```python
from build123d import *

# Parameters (mm, degrees)
SKETCH1_R                       = 12.7
BOSS_EXTRUDE1_DEPTH             = 25.4
CUT_EXTRUDE1_DEPTH              = 333.148099498
CUT_EXTRUDE1_DEPTH_BACK         = 333.148099498
SKETCH2_W                       = 25.4
SKETCH2_H                       = 50.8
BOSS_EXTRUDE2_REACH             = 334.148
SKETCH1_2_R                     = 12.7
BOSS_EXTRUDE2_DIRECTION_2_REACH = 334.148


with BuildPart() as part:
    # Sketch1 → Boss-Extrude1 (new, symmetric)
    with BuildSketch(Plane.XY):
        with BuildLine():
            Line((-25.4, 0), (-25.4, 304.8))
            ThreePointArc((-25.4, 304.8), (0, 330.2), (25.4, 304.8))
            Line((25.4, 304.8), (25.4, 0))
            ThreePointArc((25.4, 0), (0, -25.4), (-25.4, 0))
        make_face()
        Circle(SKETCH1_R, mode=Mode.SUBTRACT)
        with Locations((0, 304.8)):
            Circle(SKETCH1_R, mode=Mode.SUBTRACT)
    extrude(amount=BOSS_EXTRUDE1_DEPTH, both=True)

    # Sketch2 → Cut-Extrude1 (cut, two sides: drawn at the far end of the back side and taken through both)
    with BuildSketch(Plane(origin=(0, 0, 0), x_dir=(0, 0, -1), z_dir=(1, 0, 0)).offset(-CUT_EXTRUDE1_DEPTH_BACK)):
        with Locations((0, 304.8)):
            Rectangle(SKETCH2_W, SKETCH2_H)
        Rectangle(SKETCH2_W, SKETCH2_H)
    extrude(amount=CUT_EXTRUDE1_DEPTH + CUT_EXTRUDE1_DEPTH_BACK, mode=Mode.SUBTRACT)

    # Boss-Extrude2: up to this face of the body (flat: up to its plane)
    boss_extrude2_end = Plane(part.part.faces().sort_by_distance((0, 152.4, -25.4))[0])
    # Sketch1<2> → Boss-Extrude2 (add, up to the picked face)
    with BuildSketch(Plane.XY, mode=Mode.PRIVATE) as boss_extrude2_sk1:
        Circle(SKETCH1_2_R)
    boss_extrude2_tool1 = split(extrude(boss_extrude2_sk1.sketch, amount=-BOSS_EXTRUDE2_REACH, mode=Mode.PRIVATE), bisect_by=boss_extrude2_end, keep=Keep.BOTH, mode=Mode.PRIVATE)
    # Sketch1<2> → Boss-Extrude2 (add, up to the picked face)
    with BuildSketch(Plane.XY, mode=Mode.PRIVATE) as boss_extrude2_sk2:
        with Locations((0, 304.8)):
            Circle(SKETCH1_2_R)
    boss_extrude2_tool2 = split(extrude(boss_extrude2_sk2.sketch, amount=-BOSS_EXTRUDE2_REACH, mode=Mode.PRIVATE), bisect_by=boss_extrude2_end, keep=Keep.BOTH, mode=Mode.PRIVATE)
    add(boss_extrude2_tool1.solids().sort_by(Axis((0, 0, 0), (0, 0, -1)))[0])
    add(boss_extrude2_tool2.solids().sort_by(Axis((0, 304.8, 0), (0, 0, -1)))[0])

    # Boss-Extrude2 direction 2: up to this face of the body (flat: up to its plane)
    boss_extrude2_direction_2_end = Plane(part.part.faces().sort_by_distance((0, 152.4, 25.4))[0])
    # Sketch1<2> → Boss-Extrude2 direction 2 (add, up to the picked face)
    with BuildSketch(Plane.XY, mode=Mode.PRIVATE) as boss_extrude2_direction_2_sk1:
        Circle(SKETCH1_2_R)
    boss_extrude2_direction_2_tool1 = split(extrude(boss_extrude2_direction_2_sk1.sketch, amount=BOSS_EXTRUDE2_DIRECTION_2_REACH, mode=Mode.PRIVATE), bisect_by=boss_extrude2_direction_2_end, keep=Keep.BOTH, mode=Mode.PRIVATE)
    # Sketch1<2> → Boss-Extrude2 direction 2 (add, up to the picked face)
    with BuildSketch(Plane.XY, mode=Mode.PRIVATE) as boss_extrude2_direction_2_sk2:
        with Locations((0, 304.8)):
            Circle(SKETCH1_2_R)
    boss_extrude2_direction_2_tool2 = split(extrude(boss_extrude2_direction_2_sk2.sketch, amount=BOSS_EXTRUDE2_DIRECTION_2_REACH, mode=Mode.PRIVATE), bisect_by=boss_extrude2_direction_2_end, keep=Keep.BOTH, mode=Mode.PRIVATE)
    add(boss_extrude2_direction_2_tool1.solids().sort_by(Axis((0, 0, 0), (0, 0, 1)))[0])
    add(boss_extrude2_direction_2_tool2.solids().sort_by(Axis((0, 304.8, 0), (0, 0, 1)))[0])


solid = part.part
```
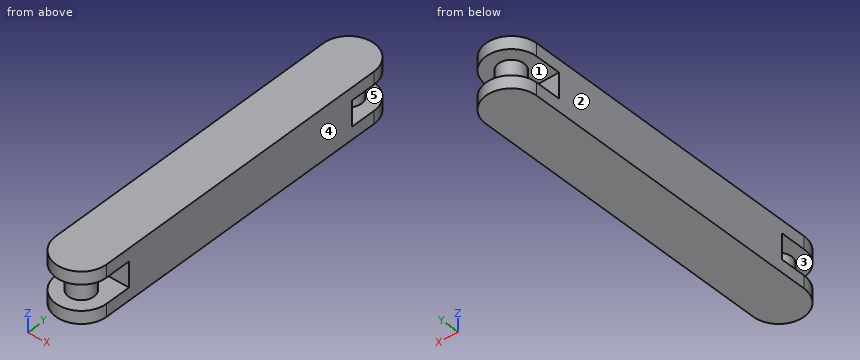
Design review of the part built by this model. Coordinates are the model's own, in mm. Face numbers are marked on the shaded views. A direction names the side the tool comes from. Round coordinates to 2 decimals unless told otherwise and drop trailing zeros. Order: outer loops, then holes, each group sorted by start corner. A loop starts at its lowest first (then second) coordinate and runs counter-clockwise, first axis right, second up. Notation, with made-up numbers: M 11,46 L 68,46 A20 ccw 68,61 Z; hole C 28,72 d10. An arc over 180 degrees is marked long. Put each result on its own line as item: value.
Q1. Consider section D-D (x = 16). State the section outline as (y, z) points.
Reported:
outline: M -19.73,-25.4 L 324.53,-25.4 L 324.53,-12.7 L 279.4,-12.7 L 279.4,12.7 L 324.53,12.7 L 324.53,25.4 L -19.73,25.4 L -19.73,12.7 L 25.4,12.7 L 25.4,-12.7 L -19.73,-12.7 Z
Q2. Consider section A-A (y = 20.5). State the section outline as (x, z) points.
Reported:
outline: M -25.4,-25.4 L 25.4,-25.4 L 25.4,-12.7 L -25.4,-12.7 Z; M -25.4,12.7 L 25.4,12.7 L 25.4,25.4 L -25.4,25.4 Z
Q3. Insertion check: pin 1 Ø8 at (x, z) = (4, 7.5) entering from +Y; pin 2 Ø6 at (x, z) = (13, 4.5) entering from +Y; pin 3 Ø3 at (x, z) = (-4, 5.5) entering from -Y. Each pin has a flat end and moves straight along its axis. Give the tip position at first contact, or say it passes through.
Reported:
pin 1: y = 317.5
pin 2: y = 312.63
pin 3: y = -12.45
Q4. Consider section B-B (x = 0). State the section outline as (y, z) points, and give its area (3 significant figures).
Reported:
outline: M -25.4,-25.4 L 330.2,-25.4 L 330.2,-12.7 L 317.5,-12.7 L 317.5,12.7 L 330.2,12.7 L 330.2,25.4 L -25.4,25.4 L -25.4,12.7 L -12.7,12.7 L -12.7,-12.7 L -25.4,-12.7 Z; hole M 12.7,-12.7 L 25.4,-12.7 L 25.4,12.7 L 12.7,12.7 Z; hole M 279.4,-12.7 L 292.1,-12.7 L 292.1,12.7 L 279.4,12.7 Z
area: 16,800 mm²
Q5. Consider section C-C (z = -6.5). State the section outline as (x, y) points, and give its area (3 significant figures).
Reported:
outline: M -25.4,25.4 L 25.4,25.4 L 25.4,279.4 L -25.4,279.4 Z; C 0,0 d25.4; C 0,304.8 d25.4
area: 13,900 mm²
Q6. To check wall thickness, follow line 1 (Y direction, x = -0.5, z = 8.5); line 2 (Z direction, x = 8.5, y = 21); line 3 (Y direction, x = -4, z = 1). State the ranges of each line that lie inside material, in increasing order.
Reported:
line 1: -12.69 to 12.69, 25.4 to 279.4, 292.11 to 317.49
line 2: -25.4 to -12.7, 12.7 to 25.4
line 3: -12.05 to 12.05, 25.4 to 279.4, 292.75 to 316.85
Q7. Machinability: for the marked faces 1 and 2, which of the approach directions +Z, -Z, +X, -X, +Y, -Y give a long, thin tool a straight path to every point of the face, cutting with its end or side? Answer none if there is none.
Reported:
face 1: none
face 2: +Z, -Z, -X, +Y, -Y
Q8. Draft analysis for pull direction Y (two halves, no side actions). For the marked faces 3, 4 and 5, state which applies: released by +Y, released by -Y, zero draft, split by the parting line, or undercut.
Reported:
face 3: undercut
face 4: zero draft
face 5: undercut
